Can you work these out from the drawing? Everything is in mm from the part's minimum corner. Round coordinates to 2 decimals unless told otherwise and drop trailing zeros. Loops run counter-clockwise (first coordinate to the right, second up) from the corner with the lowest first, then second, coordinate; pieces in that order, holes last. Notation, with made-up numbers: M 35.5,6 L 46.5,6 A24 cw 46.5,31 Z; hole C 54,20.25 d2. An arc over 180 degrees is marked long. Return JSON: item names as keys, results as strings. Group by question number.
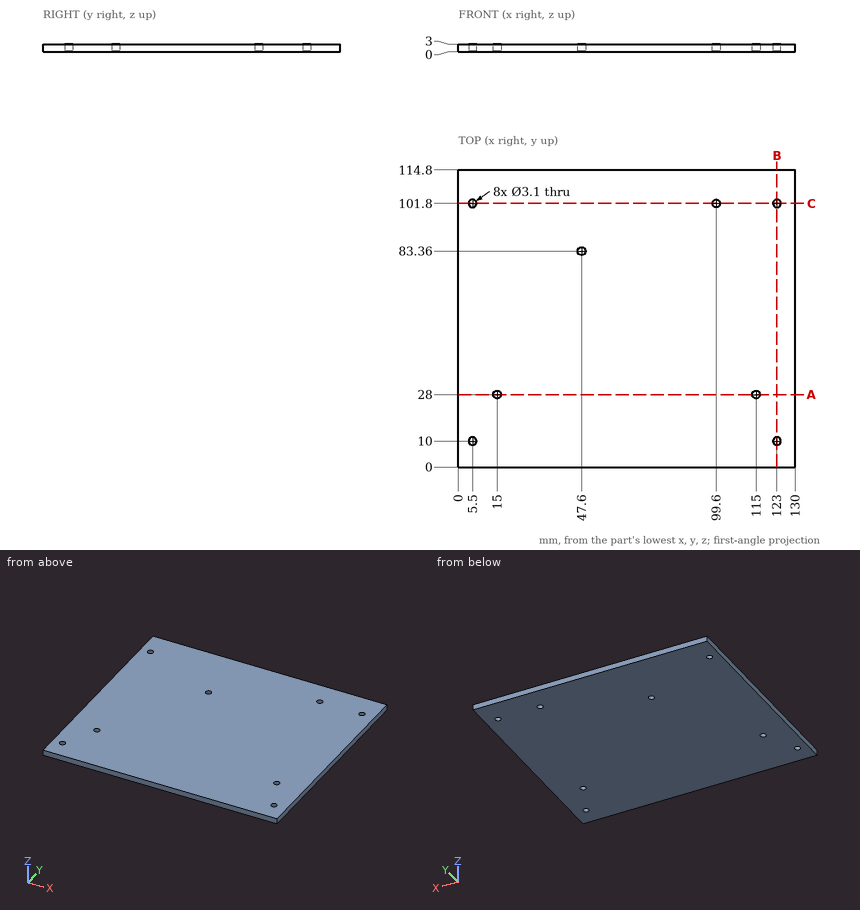
1. If we section it at B-B, the plane x = 123: Please give me the cut outline in (y, z).
2. If we section it at A-A, the plane y = 28: Please give me the cut outline in (x, z), then the cut area to 3 significant figures.
3. I need wall thicknesses on probe 1 along Y at (x, z) = (123, 1); probe 2 along Y at (x, z) = (99.6, 2.3); probe 3 along X at (y, z) = (83.36, 2.05). Which ranges of each line are inside material? Lowest first, please.
4. If we section it at C-C, the plane y = 101.8: Please give me the cut outline in (x, z), then the cut area to 3 significant figures.
5. I'm going to push flat-ended pins straight in: pin 1 Ø1.5 at (x, y) = (17, 43) entering from -Z; pin 2 Ø1.9 at (x, y) = (5.5, 10) entering from -Z. Where does each tip first touch, or does it pass through?
Geometry results:
{
 "1": {"outline": "M 0,0 L 8.45,0 L 8.45,3 L 0,3 Z; M 11.55,0 L 100.25,0 L 100.25,3 L 11.55,3 Z; M 103.35,0 L 114.8,0 L 114.8,3 L 103.35,3 Z"},
 "2": {"outline": "M 0,0 L 13.45,0 L 13.45,3 L 0,3 Z; M 16.55,0 L 113.45,0 L 113.45,3 L 16.55,3 Z; M 116.55,0 L 130,0 L 130,3 L 116.55,3 Z", "area": "371 mm^2"},
 "3": {"probe 1": "0 to 8.45, 11.55 to 100.25, 103.35 to 114.8", "probe 2": "0 to 100.25, 103.35 to 114.8", "probe 3": "0 to 46.05, 49.15 to 130"},
 "4": {"outline": "M 0,0 L 3.95,0 L 3.95,3 L 0,3 Z; M 7.05,0 L 98.05,0 L 98.05,3 L 7.05,3 Z; M 101.15,0 L 121.45,0 L 121.45,3 L 101.15,3 Z; M 124.55,0 L 130,0 L 130,3 L 124.55,3 Z", "area": "362 mm^2"},
 "5": {"pin 1": "z = 0", "pin 2": "through"}
}
